Could you check a few things on this model? Use its own coordinates, in mm. Give positions to 0.01 mm unless a question says otherwise; leave off trailing zeros. Write each loop counter-clockwise with the first axis right and the second up, starting at its lowest first coordinate (ties: lowest second). Pieces come first, ordered by that corner, then holes. Notation, with made-up numbers: (68.5, 7) - (106.5, 7) arc R12 cw to (106.5, 14) - close; hole circle Ø11 at (67, 62.25). An arc over 180 degrees is marked (long way). Write item = value, one per line.
from build123d import *

# Parameters (mm, degrees)
CHAMFER1_SIZE      = 0.22
CHAMFER1_SIZE2     = 0.381051178
CUT_EXTRUDE1_DEPTH = 0.85
CUT_EXTRUDE1_TAPER = 6


with BuildPart() as part:
    # Sketch1 → Revolve1 (revolve)
    with BuildSketch(Plane.XY, mode=Mode.PRIVATE) as revolve1_sk:
        with BuildLine():
            Line((0, 2), (-0.897999199, 2))
            ThreePointArc((-0.897999199, 2), (-1.419403703, 1.059811908), (-1.6, 0))
            Line((-1.6, 0), (9.5, 0))
            Line((9.5, 0), (9.5, 1.1))
            Line((9.5, 1.1), (0, 1.1))
            Line((0, 1.1), (0, 2))
        make_face()
    revolve(revolve1_sk.sketch.rotate(Axis((0, 0, 0), (1, 0, 0)), 90), axis=Axis((0, 0, 0), (1, 0, 0)))

    # Chamfer1
    chamfer1_edges = [part.edges().sort_by_distance(p)[0] for p in [
        (9.5, 0, -1.1),
    ]]
    chamfer1_side = [part.faces().sort_by_distance(p)[0] for p in [
        (9.5, 0, 0),
    ]]
    chamfer(chamfer1_edges, length=CHAMFER1_SIZE, length2=CHAMFER1_SIZE2, reference=chamfer1_side[0])

    # Sketch2 → EndCone (revolve, cut)
    with BuildSketch(Plane.XY, mode=Mode.PRIVATE) as endcone_sk:
        Polygon((9.5, 0), (7.594744112, 1.1), (7.594744112, 1.2), (9.6, 1.2), (9.6, 0), align=None)
    revolve(endcone_sk.sketch.rotate(Axis((0, 0, 0), (1, 0, 0)), 90), axis=Axis((0, 0, 0), (1, 0, 0)), mode=Mode.SUBTRACT)

    # Sketch3 → Cut-Extrude1 (cut)
    with BuildSketch(Plane(origin=(-1.6, 0, 0), x_dir=(0, 0, -1), z_dir=(1, 0, 0))):
        Polygon((-0.2375, 0.95), (-0.1425, 0.57), (-0.29897586, 0.29897586), (-0.57, 0.1425), (-0.95, 0.2375), (-0.95, -0.2375), (-0.57, -0.1425), (-0.29897586, -0.29897586), (-0.1425, -0.57), (-0.2375, -0.95), (0.2375, -0.95), (0.1425, -0.57), (0.29897586, -0.29897586), (0.57, -0.1425), (0.95, -0.2375), (0.95, 0.2375), (0.57, 0.1425), (0.29897586, 0.29897586), (0.1425, 0.57), (0.2375, 0.95), align=None)
    extrude(amount=CUT_EXTRUDE1_DEPTH, taper=CUT_EXTRUDE1_TAPER, mode=Mode.SUBTRACT)


solid = part.part
1. I need wall thicknesses on line 1 (X direction, y = 1.2, z = -1.55); line 2 (Z direction, x = -1, y = -1.5); line 3 (X direction, y = 1.5, z = 0.85). Which ranges of each line are inside material? Lowest first, please.
Filled sheet:
line_1 = -0.93 to 0
line_2 = -1.11 to 1.11
line_3 = -1.1 to 0
2. If we section it at A-A, the plane x = 3.5: Please give me the cut outline in (y, z), and give its area (3 significant figures).
Filled sheet:
outline = circle Ø2.2 at (0, 0)
area = 3.80 mm2
3. If we section it at B-B, the plane z = -1.6: Please give me the cut outline in (x, y).
Filled sheet:
outline = (-0.9, -1.2) - (0, -1.2) - (0, 1.2) - (-0.9, 1.2) arc R2.77 ccw to start
4. Thinking about a two-plate mould opening in Y: for faces 1 (the face through (-0.75, 0, 0)), 2 (the face through (-0.455, 1.952, -0.434)), 3 (the face through (0, 1, -1)), which applies, pulls with the +Y half, pulls with the -Y half, needs draft (parallel to the pull), parting line crosses it, or undercut?
Filled sheet:
face_1 = undercut
face_2 = parting line crosses it
face_3 = needs draft
5. If we section it at C-C, the plane y = -1.65: Please give me the cut outline in (x, z).
Filled sheet:
outline = (-0.9, -1.13) - (0, -1.13) - (0, 1.13) - (-0.9, 1.13) arc R2.74 ccw to start
6. For pin 1 (2 mm diameter, centred on x = 5, y = 1.5, fed in from -Z); pin 2 (1.5 mm diameter, centred on x = 5, y = 1, fed in from +Z); pin 3 (1.5 mm diameter, centred on x = 5.5, y = 0, fed in from -Z), each with a flat end and sliding along its axis, tell me the tip position at first contact or that it passes through.
Filled sheet:
pin_1 = -0.98
pin_2 = 1.07
pin_3 = -1.1
